Part print with two shaded views. Sizes in mm from the minimum x, y, z corner. A direction names the side the tool comes from. Coordinates: 2 decimals unless noted, no trailing zeros. Loops run counter-clockwise (first coordinate to the right, second up) from the corner with the lowest first, then second, coordinate; pieces in that order, holes last. Notation, with made-up numbers: (-4.5, 86) -> (37.5, 86) arc R17 ccw to (37.5, 93) -> close; hole circle Ø1 at (84, 85). An arc over 180 degrees is marked (long way). Return JSON: item names as keys, results as strings. Group by question number.
(1) Flat gauge pins, fed straight in: pin 1 Ø3 at (x, y) = (20.5, 4.5) entering from +Z; pin 2 Ø3 at (x, y) = (26.5, 13.5) entering from -Z. Where does each tip first touch, or does it go through?
(2) Saw through at B-B on y = 15.75. Write the cut outline in (x, z), then the cut area to 3 significant figures.
(3) Saw through at C-C on z = 5. Write the cut outline in (x, y).
(4) Tool access for the marked faces 1, 2 and 3: list every direction of +Z, -Z, +X, -X, +Y, -Y with a clear straight run to the whole face (end or side of a thin tool).
(5) Probe L1, parallel to Y at x = 2.25, z = 7; L2, parallel to X at y = 14.5, z = 9.25; L3, parallel to Y at x = 8, z = 2.25. List the from-to ranges inside material, lowest first.
(6) Saw through at A-A on x = 2.25. Write the cut outline in (y, z).
(7) Mould opens along X. For the marked faces 4, 5, 6 and 7 say: pulls with the +X half, pulls with the -X half, needs draft (parallel to the pull), parting line crosses it, or undercut.
(8) Saw through at D-D on x = 17.75. Write the cut outline in (y, z), then the cut area to 3 significant figures.
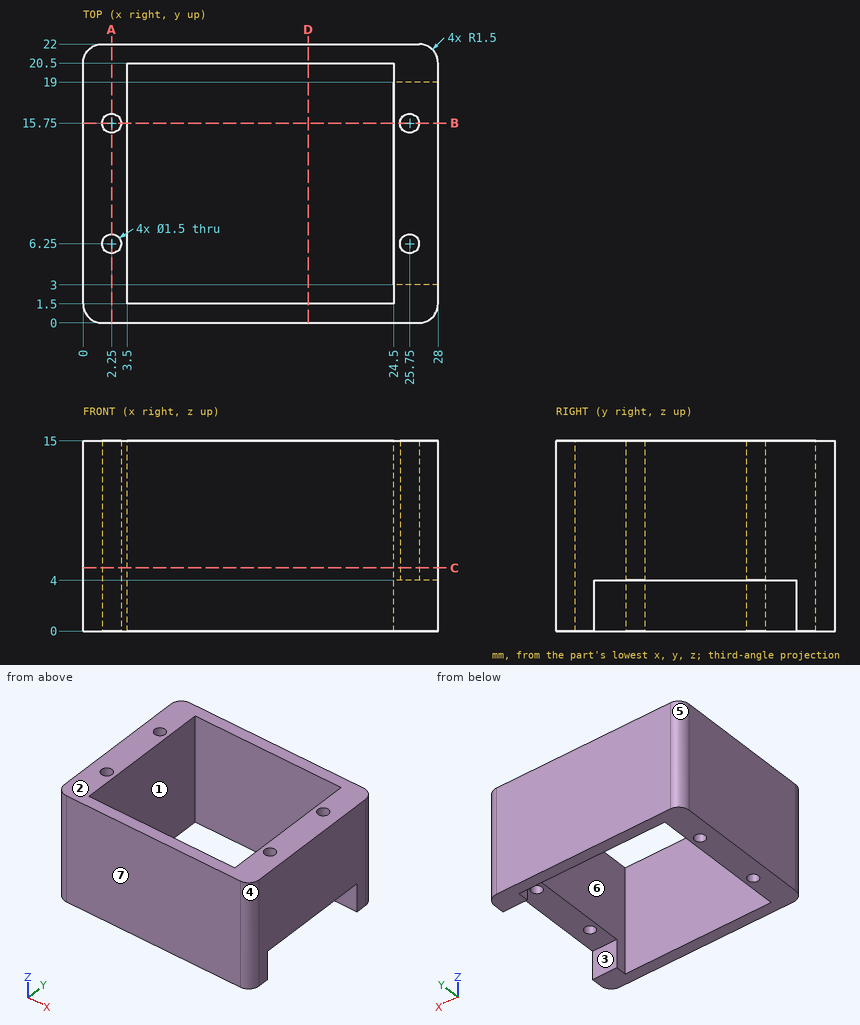
Geometry results:
{
 "1": {"pin 1": "through", "pin 2": "z = 4"},
 "2": {"outline": "(0, 0) -> (1.5, 0) -> (1.5, 15) -> (0, 15) -> close; (3, 0) -> (3.5, 0) -> (3.5, 15) -> (3, 15) -> close; (24.5, 4) -> (25, 4) -> (25, 15) -> (24.5, 15) -> close; (26.5, 4) -> (28, 4) -> (28, 15) -> (26.5, 15) -> close", "area": "52.0 mm²"},
 "3": {"outline": "(0, 1.5) arc R1.5 ccw to (1.5, 0) -> (26.5, 0) arc R1.5 ccw to (28, 1.5) -> (28, 20.5) arc R1.5 ccw to (26.5, 22) -> (1.5, 22) arc R1.5 ccw to (0, 20.5) -> close; hole circle Ø1.5 at (2.25, 6.25); hole circle Ø1.5 at (2.25, 15.75); hole (3.5, 1.5) -> (24.5, 1.5) -> (24.5, 20.5) -> (3.5, 20.5) -> close; hole circle Ø1.5 at (25.75, 6.25); hole circle Ø1.5 at (25.75, 15.75)"},
 "4": {"face 1": "+Z, -Z", "face 2": "+Z, +X, -X, +Y, -Y", "face 3": "-Z, +X"},
 "5": {"L1": "0 to 5.5, 7 to 15, 16.5 to 22", "L2": "0 to 3.5, 24.5 to 28", "L3": "0 to 1.5, 20.5 to 22"},
 "6": {"outline": "(0, 0) -> (5.5, 0) -> (5.5, 15) -> (0, 15) -> close; (7, 0) -> (15, 0) -> (15, 15) -> (7, 15) -> close; (16.5, 0) -> (22, 0) -> (22, 15) -> (16.5, 15) -> close"},
 "7": {"face 4": "pulls with the +X half", "face 5": "pulls with the -X half", "face 6": "undercut", "face 7": "needs draft"},
 "8": {"outline": "(0, 0) -> (1.5, 0) -> (1.5, 15) -> (0, 15) -> close; (20.5, 0) -> (22, 0) -> (22, 15) -> (20.5, 15) -> close", "area": "45.0 mm²"}
}
